```python
from build123d import *

# Parameters (mm, degrees)
CROQUIS1_R              = 13.7
SALIENTE_EXTRUIR1_DEPTH = 5
CROQUIS2_R              = 9.5
CORTAR_EXTRUIR1_DEPTH   = 3.5
CROQUIS3_R              = 6.8
CORTAR_EXTRUIR2_DEPTH   = 3
SALIENTE_EXTRUIR2_START = 2
CROQUIS4_R              = 13.7
CROQUIS4_R_2            = 6.65
SALIENTE_EXTRUIR2_DEPTH = 2
CROQUIS5_R              = 1.25
CORTAR_EXTRUIR3_DEPTH   = 21.600485431


with BuildPart() as part:
    # Croquis1 → Saliente-Extruir1 (new body)
    with BuildSketch(Plane.XY):
        Circle(CROQUIS1_R)
        with BuildLine():
            Line((0, 0.75), (7.800197377, 0.75))
            ThreePointArc((7.800197377, 0.75), (10.459785271, 2.369760146), (12.48, 0))
            ThreePointArc((12.48, 0), (10.459785271, -2.369760146), (7.800197377, -0.75))
            Line((7.800197377, -0.75), (0, -0.75))
            Line((0, -0.75), (-7.800197377, -0.75))
            ThreePointArc((-7.800197377, -0.75), (-12.48, 0), (-7.800197377, 0.75))
            Line((-7.800197377, 0.75), (0, 0.75))
        make_face(mode=Mode.SUBTRACT)
    extrude(amount=SALIENTE_EXTRUIR1_DEPTH)

    # Croquis2 → Cortar-Extruir1 (cut)
    with BuildSketch(Plane.XY.offset(5)):
        Circle(CROQUIS2_R)
    extrude(amount=-CORTAR_EXTRUIR1_DEPTH, mode=Mode.SUBTRACT)

    # Croquis3 → Cortar-Extruir2 (cut)
    with BuildSketch(Plane.XY.offset(1.5)):
        Circle(CROQUIS3_R)
    extrude(amount=-CORTAR_EXTRUIR2_DEPTH, mode=Mode.SUBTRACT)

    # Croquis4 → Saliente-Extruir2 (add)
    with BuildSketch(Plane(origin=(0, 0, 0), x_dir=(-1, 0, 0), z_dir=(0, 0, -1)).offset(SALIENTE_EXTRUIR2_START)):
        Circle(CROQUIS4_R)
        Circle(CROQUIS4_R_2, mode=Mode.SUBTRACT)
    extrude(amount=-SALIENTE_EXTRUIR2_DEPTH)

    # Croquis5 → Cortar-Extruir3 (cut, through all)
    with BuildSketch(Plane.XY.offset(5)):
        with Locations((-10.08, 0)):
            Circle(CROQUIS5_R)
        with Locations((10.08, 0)):
            Circle(CROQUIS5_R)
    extrude(amount=-CORTAR_EXTRUIR3_DEPTH, mode=Mode.SUBTRACT)


solid = part.part
```
Part model, mm, in its own coordinate system. A direction names the side the tool comes from. Coordinates: 2 decimals unless noted, no trailing zeros. Write each loop counter-clockwise with the first axis right and the second up, starting at its lowest first coordinate (ties: lowest second). Pieces come first, ordered by that corner, then holes.
Item 1: Slice it at C-C (y = -5.75). Write the cut outline in (x, z), and give its area (3 significant figures).
Item 2: Probe line 1 (Y direction, x = 0, z = -0.65); line 2 (X direction, y = 3.5, z = 0.25); line 3 (Y direction, x = -3.5, z = 3). List the from-to ranges inside material, lowest first.
Item 3: Which spindle directions (+Z, -Z, +X, -X, +Y, -Y) get a long thin tool onto all of the face, cutting with end or side? Do faces 1 (the face through (11.27, 0.38, -0.99)), 2 (the face through (-0.1, -6.8, 0.8)). Say none if no direction does.
Item 4: Slice it at D-D (z = -1). Write the cut outline in (x, y), and give its area (3 significant figures).
Item 5: Slice it at A-A (x = 0). Write the cut outline in (y, z).
Item 6: Pin check, flat tips, straight feed: pin 1 (0.8 mm diameter, centred on x = -7, z = 0.5, fed in from +Y); pin 2 (1.5 mm diameter, centred on x = -10.08, y = 0, fed in from +Z); pin 3 (1.5 mm diameter, centred on x = 1.5, z = 3.5, fed in from -Y); pin 4 (1.1 mm diameter, centred on x = 7.5, z = 0.5, fed in from -Y). Stop position of each tip, or through.
Item 7: Slice it at B-B (z = 1). Write the cut outline in (x, y).
Item 8: Mould opens along Y. For faces 3 (the face through (6.3, -2.9, -2)), 4 (the face through (0, -7, 1.5)) say: released by +Y, released by -Y, zero draft, split by the parting line, or undercut.
Results found:
1. outline: (-12.43, -2) - (-3.34, -2) - (-3.34, 0) - (-3.63, 0) - (-3.63, 1.5) - (-7.56, 1.5) - (-7.56, 5) - (-12.43, 5) - close; (3.34, -2) - (12.43, -2) - (12.43, 5) - (7.56, 5) - (7.56, 1.5) - (3.63, 1.5) - (3.63, 0) - (3.34, 0) - close
1. area: 96.9 mm2
2. line 1: y = -13.7 to -6.65, 6.65 to 13.7
2. line 2: x = -13.25 to -5.83, 5.83 to 13.25
2. line 3: y = -13.25 to -8.83, 8.83 to 13.25
3. face 1: +Z, -Z
3. face 2: +Z
4. outline: circle Ø27.4 at (0, 0); hole circle Ø2.5 at (-10.08, 0); hole circle Ø13.3 at (0, 0); hole circle Ø2.5 at (10.08, 0)
4. area: 441 mm2
5. outline: (-13.7, -2) - (-6.65, -2) - (-6.65, 0) - (-6.8, 0) - (-6.8, 1.5) - (-9.5, 1.5) - (-9.5, 5) - (-13.7, 5) - close; (6.65, -2) - (13.7, -2) - (13.7, 5) - (9.5, 5) - (9.5, 1.5) - (6.8, 1.5) - (6.8, 0) - (6.65, 0) - close
6. pin 1: stops at y = 12.01
6. pin 2: passes through
6. pin 3: stops at y = -13.68
6. pin 4: stops at y = -11.81
7. outline: circle Ø27.4 at (0, 0); hole (-7.8, -0.75) - (-6.76, -0.75) arc R6.8 ccw to (6.76, -0.75) - (7.8, -0.75) arc R2.4 ccw (long way) to (7.8, 0.75) - (6.76, 0.75) arc R6.8 ccw to (-6.76, 0.75) - (-7.8, 0.75) arc R2.4 ccw (long way) to start
8. face 3: zero draft
8. face 4: undercut
